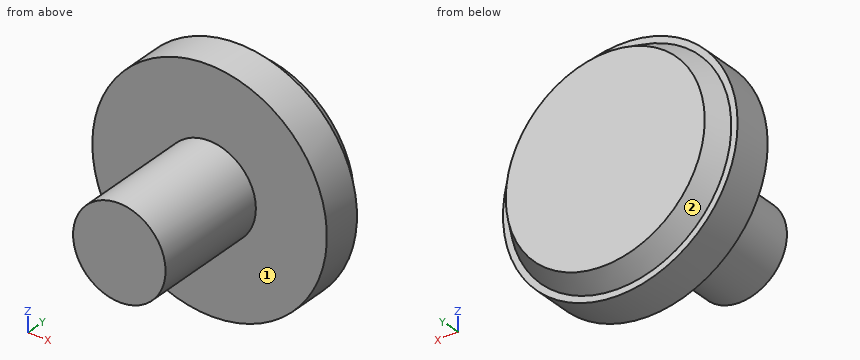
Autodesk Inventor part; units mm, degrees
ref_plane "YZ Plane" through (0, 0, 0) normal (1, 0, 0) x (0, 1, 0)
ref_plane "XZ Plane" through (0, 0, 0) normal (0, 1, 0) x (-1, 0, 0)
ref_plane "XY Plane" through (0, 0, 0) normal (0, 0, 1) x (1, 0, 0)
sketch "Sketch1" plane through (0, 0, 0) normal (0, 1, 0) x (-1, 0, 0)
  line L0 (0, -41.9252) -> (0, 41.9252)
  line L1 (-41.9252, 0) -> (41.9252, 0)
  circle A0 centre (0, 0) radius 29.9466
  dimension "d0" = 59.8932
extrude "Extrusion1" add sketch "Sketch1" along normal blind 10.16
sketch "Sketch2" plane through (0, 0, 0) normal (0, 0, 1) x (1, 0, 0)
  line L0 (-29.9466, 0) -> (29.9466, 0)
  line L1 (29.9466, 10.16) -> (-29.9466, 10.16)
  line L2 (-29.9466, 0) -> (0, 0)
  line L3 (0, 0) -> (0, 10.16)
  line L4 (0, 10.16) -> (-29.9466, 10.16)
  line L5 (-29.9466, 10.16) -> (-29.9466, 0)
  line L6 (-29.9466, 0) -> (-27.4066, 10.16)
  line L7 (-29.9466, 10.16) -> (-27.4066, 10.16)
  dimension "d4" = 2.54
sketch "Sketch3" plane through (0, 10.16, 0) normal (0, 1, 0) x (1, 0, 0)
  circle A0 centre (0, 0) radius 25.4
  dimension "d8" = 50.8
extrude "Extrusion2" add sketch "Sketch3" along normal blind 5.08
draft "FaceDraft1" angle -30 pull direction (0, -1, 0) faces at (25.3176, 13.5467, 2.0439) fixed edges at (-25.4, 15.24, 0)
sketch "Sketch4" plane through (0, 0, 0) normal (0, -1, 0) x (1, 0, 0)
  circle A0 centre (0, 0) radius 11.811
  dimension "d9" = 23.622
extrude "Extrusion3" add sketch "Sketch4" along normal blind 30.48
properties part number "ButtonLarge"
CAD build for the part. Positions are in the model's coordinates, mm. Face numbers are marked on the shaded views. A direction names the side the tool comes from. Round coordinates to 2 decimals unless told otherwise and drop trailing zeros. Order: outer loops, then holes, each group sorted by start corner. A loop starts at its lowest first (then second) coordinate and runs counter-clockwise, first axis right, second up. Notation, with made-up numbers: (70, 58) -> (88, 58) arc R26 ccw to (88, 78) -> close; hole circle Ø2 at (11, -6). An arc over 180 degrees is marked (long way). One line per question, with ' | ' between items.
Q1. Slice it at B-B (x = 0). Write the cut outline in (y, z), then the cut area to 3 significant figures.
Completed:
outline: (-30.48, -11.81) -> (0, -11.81) -> (0, -29.95) -> (10.16, -29.95) -> (10.16, -28.33) -> (15.24, -25.4) -> (15.24, 25.4) -> (10.16, 28.33) -> (10.16, 29.95) -> (0, 29.95) -> (0, 11.81) -> (-30.48, 11.81) -> close | area: 1,600 mm^2
Q2. Which spindle directions (+Z, -Z, +X, -X, +Y, -Y) get a long thin tool onto all of the face, cutting with end or side? Do the marked faces 1 and 2. Say none if no direction does.
Completed:
face 1: -Y | face 2: +Y
Q3. Drop flat-ended pins along their axis: pin 1 (4 mm diameter, centred on y = -14, z = -8, fed in from +X); pin 2 (5 mm diameter, centred on y = -1, z = -9, fed in from +X); pin 3 (12 mm diameter, centred on y = -22, z = -19.5, fed in from +X); pin 4 (1.5 mm diameter, centred on y = 8, z = 1.5, fed in from -X). Give the stop position or say it passes through.
Completed:
pin 1: stops at x = 10.17 | pin 2: stops at x = 29.19 | pin 3: passes through | pin 4: stops at x = -29.94
Q4. Slice it at D-D (y = 2). Write the cut outline in (x, z), then the cut area to 3 significant figures.
Completed:
outline: circle Ø59.89 at (0, 0) | area: 2,820 mm^2
Q5. Probe probe 1 along Y at (x, z) = (-12.5, 21); probe 2 along Y at (x, z) = (22, -19); probe 3 along X at (y, z) = (11, -12.5). List the from-to ranges inside material, lowest first.
Completed:
probe 1: y = 0 to 15.24 | probe 2: y = 0 to 10.16 | probe 3: x = -24.88 to 24.88
Q6. Slice it at A-A (z = 0). Write the cut outline in (x, y), then the cut area to 3 significant figures.
Completed:
outline: (-29.95, 0) -> (-11.81, 0) -> (-11.81, -30.48) -> (11.81, -30.48) -> (11.81, 0) -> (29.95, 0) -> (29.95, 10.16) -> (28.33, 10.16) -> (25.4, 15.24) -> (-25.4, 15.24) -> (-28.33, 10.16) -> (-29.95, 10.16) -> close | area: 1,600 mm^2
Q7. Slice it at C-C (y = -11). Write the cut outline in (x, z).
Completed:
outline: circle Ø23.62 at (0, 0)
